from build123d import *

# Parameters (mm, degrees)
F0_R        = 3
F1_DEPTH    = 13
F2_R        = 7
F3_R        = 6.5
F4_T1_DEPTH = 13
F4_T3_DEPTH = 18.1433659759
F4_T5_DEPTH = 15.2571417204


# Not quite as in the source:
# - a fillet or chamfer that OpenCascade refuses, or shapes differently, is made with other operations: its cross-section is extruded or revolved along the edge and cut away or added


with BuildPart() as f1:
    # F0 (on Top) → F1 (new body)
    with BuildSketch(Plane.XY):
        with BuildLine():
            Line((18, 18), (0, 0))
            Line((0, 0), (-11, 11))
            ThreePointArc((-11, 11), (-12.8659446975, 12.2241130817), (-12.4367385267, 14.4140867148))
            Line((-12.4367385267, 14.4140867148), (-11, 15.8508252416))
            Line((-11, 15.8508252416), (-11, 21.9997463049))
            Line((-11, 21.9997463049), (-23, 21.9997463049))
            Line((-23, 21.9997463049), (-23, -0.1923881554))
            Line((-23, -0.1923881554), (-6.5, -16.6923881554))
            Line((-6.5, -16.6923881554), (-6.5, -96.6923881554))
            Line((-6.5, -96.6923881554), (6.5, -96.6923881554))
            Line((6.5, -96.6923881554), (6.5, -16.6923881554))
            Line((6.5, -16.6923881554), (27.1923881554, 4))
            Line((27.1923881554, 4), (27.1923881554, 18))
            Line((27.1923881554, 18), (18, 18))
        make_face()
        with Locations((20.6923881554, 11.5)):
            Circle(F0_R, mode=Mode.SUBTRACT)
    extrude(amount=F1_DEPTH)

    # F2
    f2_edges = [f1.edges().sort_by_distance(p)[0] for p in [
        (18, 18, 6.5),
    ]]
    fillet(f2_edges, radius=F2_R)

    # F3
    f3_edges = [f1.edges().sort_by_distance(p)[0] for p in [
        (27.192388, 18, 6.5),
    ]]
    fillet(f3_edges, radius=F3_R)

    # F4: chamfer of 1 on 5 edges, made by hand

    # F4_s2 → F4_t1 (join)
    with BuildSketch(Plane.XY):
        Polygon((-6.5, -17.1066017178), (-6.7928932188, -16.3994949366), (-6.5, -16.6923881554), align=None)
        Polygon((6.7928932188, -16.3994949366), (6.5, -17.1066017178), (6.5, -16.6923881554), align=None)
    extrude(amount=F4_T1_DEPTH)

    # F4_s4 → F4_t3 (cut)
    with BuildSketch(Plane.XY.offset(-2.571682988)):
        Polygon((-11, 20.9997463049), (-12, 21.9997463049), (-11, 21.9997463049), align=None)
        Polygon((-22, 21.9997463049), (-23, 20.9997463049), (-23, 21.9997463049), align=None)
    extrude(amount=F4_T3_DEPTH, mode=Mode.SUBTRACT)

    # F4_s6 → F4_t5 (cut)
    with BuildSketch(Plane.XY.offset(-1.1285708602)):
        Polygon((-22.7071067812, -0.4852813742), (-23, 0.2218254069), (-23, -0.1923881554), align=None)
    extrude(amount=F4_T5_DEPTH, mode=Mode.SUBTRACT)


solid = f1.part
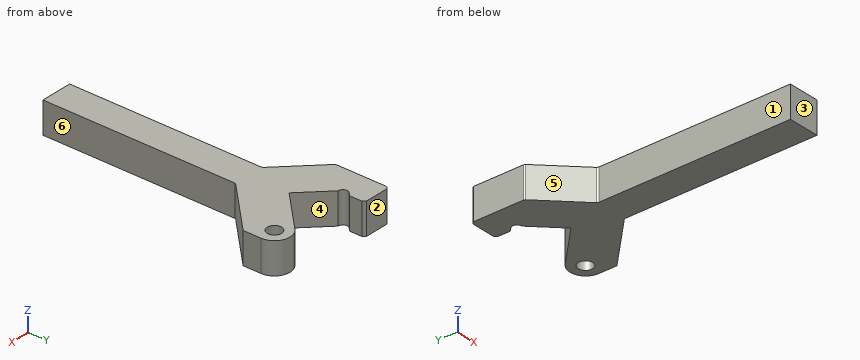
Source: CAD feature listing. Evaluate the final solid. Frame: model axes, mm. Face numbers are marked on the shaded views. A direction names the side the tool comes from. Round coordinates to 2 decimals unless told otherwise and drop trailing zeros. Loops run counter-clockwise (first coordinate to the right, second up) from the corner with the lowest first, then second, coordinate; pieces in that order, holes last. Notation, with made-up numbers: (32.5, 0) - (43.5, 0) arc R13 ccw to (43.5, 8) - close; hole circle Ø9 at (25, 15.5). An arc over 180 degrees is marked (long way). Write item = value, one per line. Start each with the question number.
Item 1: Mould query, pull axis Y, two halves, no side actions, for the marked faces 1, 2 and 3. Classes: released by +Y, released by -Y, zero draft, split by the parting line, or undercut.
Item 2: Section query A-A on y = -76.5. Output: boundary loops of the cut face in (x, z), plus the area to 3 significant figures.
Item 3: First-contact query: pin 1 Ø5 at (x, y) = (20.69, 11.5) entering from +Z; pin 2 Ø6 at (x, z) = (11, 8.5) entering from +Y; pin 3 Ø1.5 at (y, z) = (-30, 4) entering from +X; pin 4 Ø4 at (y, z) = (-32, 8) entering from -X. Flat tips, straight axial feed; report the tip coordinate or a pass-through.
Item 4: Reachability of the marked faces 4, 5 and 6 from +Z, -Z, +X, -X, +Y, -Y: full face, straight path, thin tool, end or side. Return the list, or none.
Item 5: Section query B-B on x = -4.5. Output: boundary loops of the cut face in (y, z).
Item 6: Material intervals for line 1 (Y direction, x = 0, z = 11); line 2 (X direction, y = -87.5, z = 5.5); line 3 (X direction, y = 6, z = 1.25), sorted ascending.
Results list:
q1.face_1 = zero draft
q1.face_2 = released by +Y
q1.face_3 = released by -Y
q2.outline = (-6.5, 0) - (6.5, 0) - (6.5, 13) - (-6.5, 13) - close
q2.area = 169 mm²
q3.pin_1 = through
q3.pin_2 = 14
q3.pin_3 = 6.5
q3.pin_4 = -6.5
q4.face_4 = +Z, -Z, +Y
q4.face_5 = +Z, -Z, -X, -Y
q4.face_6 = +Z, -Z, +X, -Y
q5.outline = (-96.69, 0) - (4.5, 0) - (4.5, 13) - (-96.69, 13) - close
q6.line_1 = -96.69 to 0
q6.line_2 = -6.5 to 6.5
q6.line_3 = -23 to -6, 6 to 27.19
